```python
from build123d import *

# Parameters (mm, degrees)
SKETCH1_R           = 7.5
BOSS_EXTRUDE1_DEPTH = 3
SKETCH2_R           = 5
BOSS_EXTRUDE2_DEPTH = 14
BOSS_EXTRUDE2_TAPER = -5
SKETCH4_R           = 6.5
CUT_EXTRUDE1_DEPTH  = 2
SKETCH5_R           = 5.5
CUT_EXTRUDE2_DEPTH  = 14
CUT_EXTRUDE2_TAPER  = 5
FILLET1_R           = 0.5
FILLET2_R           = 0.5
BOSS_EXTRUDE3_DEPTH = 0.05


with BuildPart() as part:
    # Sketch1 → Boss-Extrude1 (new body)
    with BuildSketch(Plane(origin=(0, 0, 0), x_dir=(1, 0, 0), z_dir=(0, 1, 0))):
        Circle(SKETCH1_R)
    extrude(amount=BOSS_EXTRUDE1_DEPTH)

    # Sketch2 → Boss-Extrude2 (add)
    with BuildSketch(Plane(origin=(0, 17, 0), x_dir=(1, 0, 0), z_dir=(0, 1, 0))):
        Circle(SKETCH2_R)
    extrude(amount=-BOSS_EXTRUDE2_DEPTH, taper=BOSS_EXTRUDE2_TAPER)

    # Sketch4 → Cut-Extrude1 (cut)
    with BuildSketch(Plane.XZ):
        Circle(SKETCH4_R)
    extrude(amount=-CUT_EXTRUDE1_DEPTH, mode=Mode.SUBTRACT)

    # Sketch5 → Cut-Extrude2 (cut)
    with BuildSketch(Plane.XZ.offset(-2)):
        Circle(SKETCH5_R)
    extrude(amount=-CUT_EXTRUDE2_DEPTH, taper=CUT_EXTRUDE2_TAPER, mode=Mode.SUBTRACT)

    # Fillet1
    fillet1_edges = [part.edges().sort_by_distance(p)[0] for p in [
        (-7.5, 3, 0),
    ]]
    fillet(fillet1_edges, radius=FILLET1_R)

    # Fillet2
    fillet2_edges = [part.edges().sort_by_distance(p)[0] for p in [
        (-5, 17, 0),
    ]]
    fillet(fillet2_edges, radius=FILLET2_R)

    # Sketch7 → Boss-Extrude3 (add)
    with BuildSketch(Plane(origin=(0, 17, 0), x_dir=(1, 0, 0), z_dir=(0, 1, 0))):
        Polygon((-0.372418319, -0.372418319), (0.334688462, 0.334688462), (-2.876818043, 3.546194967), (-3.583924824, 2.839088186), align=None)
    extrude(amount=BOSS_EXTRUDE3_DEPTH)


solid = part.part
```
The model under review builds one solid part; all positions refer to its coordinate system, in mm. A direction names the side the tool comes from. Round coordinates to 2 decimals unless told otherwise and drop trailing zeros. Loops run counter-clockwise (first coordinate to the right, second up) from the corner with the lowest first, then second, coordinate; pieces in that order, holes last.
Item 1: For faces 4 (the face through (0, 16, 0)), 5 (the face through (-1.5, 17.05, -1.6)), 6 (the face through (0, 17, 1)), list the 3-axis set-ups (+Z, -Z, +X, -X, +Y, -Y) from which the entire face can be reached by the end or side of a thin tool; tool diameter is ignored.
Determined:
face 4: -Y
face 5: +Z, -Z, +X, -X, +Y
face 6: +Y
Item 2: Take a section at A-A (y = 10). Write out the cut boundary in (x, z).
Determined:
outline: circle Ø11.22 at (0, 0); hole circle Ø9.6 at (0, 0)
Item 3: For line 1 (Z direction, x = 0, y = 0.9); line 2 (Y direction, x = -5.75, z = 2.5); line 3 (Y direction, x = 0, z = 3.75), list the stretches that pass through material, from the lowest coordinate up.
Determined:
line 1: z = -7.5 to -6.5, 6.5 to 7.5
line 2: y = 2 to 3
line 3: y = 16 to 17
Item 4: Clearance check with flat-ended pins moving along their axes: pin 1 Ø4.5 at (x, z) = (-1, 0) entering from -Y; pin 2 Ø6 at (x, y) = (1.5, 8.5) entering from +Z; pin 3 Ø3 at (x, y) = (-1.5, 14) entering from +Z. State where each tip first meets the part, or that it passes through.
Determined:
pin 1: stops at y = 16
pin 2: stops at z = 5.98
pin 3: stops at z = 5.34
Item 5: Take a section at B-B (x = 0). Write out the cut boundary in (y, z).
Determined:
outline: (0, -7.5) - (2.5, -7.5) arc R0.5 ccw to (3, -7) - (3, -6.22) - (16.54, -5.04) arc R0.5 ccw to (17, -4.54) - (17, -0.67) - (17.05, -0.67) - (17.05, 0) - (17, 0) - (17, 4.54) arc R0.5 ccw to (16.54, 5.04) - (3, 6.22) - (3, 7) arc R0.5 ccw to (2.5, 7.5) - (0, 7.5) - (0, 6.5) - (2, 6.5) - (2, 5.5) - (16, 4.28) - (16, -4.28) - (2, -5.5) - (2, -6.5) - (0, -6.5) - close
Item 6: Mouldability with a two-part tool opening along X and no side actions: class faces 1 (the face through (-5.158, 0.986, -3.955)), 2 (the face through (-5, 3, 4)), 3 (the face through (-7.493, 1.232, -0.33)) as released by +X, released by -X, zero draft, split by the parting line, or undercut.
Determined:
face 1: undercut
face 2: zero draft
face 3: split by the parting line
Item 7: Take a section at C-C (y = 7.75). Write out the cut boundary in (x, z).
Determined:
outline: circle Ø11.62 at (0, 0); hole circle Ø9.99 at (0, 0)
